Here's how the part is built. I have some questions about the finished solid (model axes, mm). Face numbers are marked on the shaded views. A direction names the side the tool comes from. Round coordinates to 2 decimals unless told otherwise and drop trailing zeros. Order: outer loops, then holes, each group sorted by start corner. A loop starts at its lowest first (then second) coordinate and runs counter-clockwise, first axis right, second up. Notation, with made-up numbers: (28.25, 74.25) - (74.25, 74.25) arc R15 ccw to (74.25, 82.25) - close; hole circle Ø3 at (20.25, -6.75). An arc over 180 degrees is marked (long way). One line per item, written item: value.
Autodesk Inventor part; units mm, degrees
ref_plane "YZ Plane" through (0, 0, 0) normal (1, 0, 0) x (0, 1, 0)
ref_plane "XZ Plane" through (0, 0, 0) normal (0, 1, 0) x (-1, 0, 0)
ref_plane "XY Plane" through (0, 0, 0) normal (0, 0, 1) x (1, 0, 0)
sketch "Sketch1" plane through (0, 0, 0) normal (0, 0, 1) x (1, 0, 0)
  line L0 (0, 0) -> (16.5, 0)
  line L1 (16.5, 0) -> (16.5, -24)
  line L2 (16.5, -24) -> (0, -24)
  line L3 (0, -24) -> (0, 0)
  line L4 (24.2611, -12.002) -> (-7.0214, -12.002)
  line L5 (10.5138, 0) -> (10.5138, -25.2396)
  line L6 (10.5138, -12.002) -> (10.5138, -20.002) construction
  line L7 (10.5138, -12.002) -> (10.5138, -4.002) construction
  circle A0 centre (10.5138, -4.002) radius 2
  circle A1 centre (10.5138, -20.002) radius 2
  circle A2 centre (4.1138, -12.002) radius 2
  dimension "d0" = 16.5
  dimension "d1" = 24
  dimension "d2" = 8
  dimension "d3" = 8
  dimension "d4" = 4
  dimension "d5" = 4
  dimension "d7" = 4
extrude "Extrusion1" add sketch "Sketch1" along normal blind 3 contours L0 L5 A0 L4 A2 L3 | L0 L1 L4 L5 A0 | L4 A2 L5 A1 L2 L3 | L1 L2 L5 A1 L4
sketch "Sketch3" plane through (16.5, -24, 0) normal (1, 0, 0) x (0, 0, -1)
  line L0 (0, 0) -> (-9, 0)
  line L1 (-9, 0) -> (-9, 24)
  line L2 (-9, 24) -> (0, 24)
  line L3 (0, 24) -> (0, 0)
  dimension "d17" = 9
extrude "Extrusion3" add sketch "Sketch3" along normal blind 3
properties part number "bart y clips"
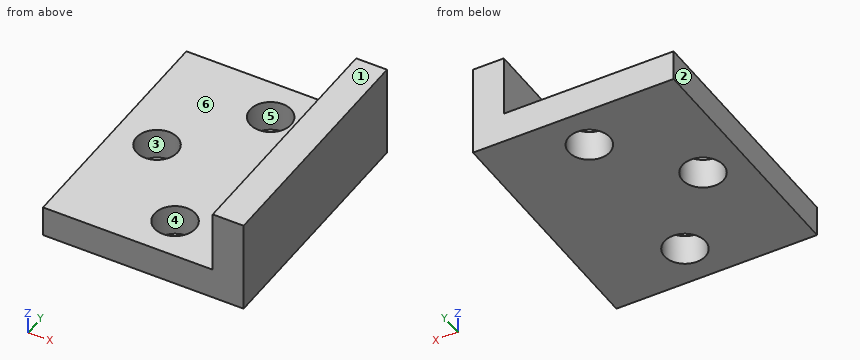
Q1. If we section it at D-D, the plane x = 11.75: Please give me the cut outline in (y, z).
Results list:
outline: (-24, 0) - (-21.57, 0) - (-21.57, 3) - (-24, 3) - close; (-18.43, 0) - (-5.57, 0) - (-5.57, 3) - (-18.43, 3) - close; (-2.43, 0) - (0, 0) - (0, 3) - (-2.43, 3) - close
Q2. Will these pins go through, and if not, where does the flat tip stop? pin 1 (6.5 mm diameter, centred on x = 10.51, y = -4, fed in from +Z); pin 2 (5 mm diameter, centred on y = -18.5, z = 6, fed in from -X); pin 3 (6.5 mm diameter, centred on x = 4.11, y = -12, fed in from -Z).
Results list:
pin 1: z = 3
pin 2: x = 16.5
pin 3: z = 0
Q3. If we section it at A-A, the plane x = 5.25: Please give me the cut outline in (y, z), then the cut area to 3 significant figures.
Results list:
outline: (-24, 0) - (-13.65, 0) - (-13.65, 3) - (-24, 3) - close; (-10.36, 0) - (0, 0) - (0, 3) - (-10.36, 3) - close
area: 62.1 mm²
Q4. If I drill on line 1 along Z through (x, y) = (14.75, -2.5); line 2 along X through (y, z) = (-12.25, 6.25); line 3 along Y through (x, z) = (5, 1), over which ranges is the centre line in solid material (lowest first)?
Results list:
line 1: 0 to 3
line 2: 16.5 to 19.5
line 3: -24 to -13.79, -10.21 to 0
Q5. We'd pull the mould along X, two halves only. Please class the marked faces 1, 2, 3 and 4: released by +X, released by -X, zero draft, split by the parting line, or undercut.
Results list:
face 1: zero draft
face 2: released by -X
face 3: undercut
face 4: undercut
Q6. If we section it at B-B, the plane y = -19.5: Please give me the cut outline in (x, z).
Results list:
outline: (0, 0) - (8.58, 0) - (8.58, 3) - (0, 3) - close; (12.45, 0) - (19.5, 0) - (19.5, 9) - (16.5, 9) - (16.5, 3) - (12.45, 3) - close
Q7. If we section it at C-C, the plane z = 2: Please give me the cut outline in (x, y), then the cut area to 3 significant figures.
Results list:
outline: (0, -24) - (19.5, -24) - (19.5, 0) - (0, 0) - close; hole circle Ø4 at (4.11, -12); hole circle Ø4 at (10.51, -20); hole circle Ø4 at (10.51, -4)
area: 430 mm²
Q8. Which directions (+Z, -Z, +X, -X, +Y, -Y) give clear straight access to the entire face, cutting with the end or side of a thin tool? Please do the marked faces 5 and 6.
Results list:
face 5: +Z, -Z
face 6: +Z, -X, +Y, -Y
